Source: CAD feature listing. Evaluate the final solid. Frame: model axes, mm. Face numbers are marked on the shaded views. Coordinates: 2 decimals unless noted, no trailing zeros. Order: outer loops, then holes, each group sorted by start corner. A loop starts at its lowest first (then second) coordinate and runs counter-clockwise, first axis right, second up.
Autodesk Inventor part; units mm, degrees
ref_plane "YZ Plane" through (0, 0, 0) normal (1, 0, 0) x (0, 1, 0)
ref_plane "XZ Plane" through (0, 0, 0) normal (0, 1, 0) x (-1, 0, 0)
ref_plane "XY Plane" through (0, 0, 0) normal (0, 0, 1) x (1, 0, 0)
sketch "Sketch1" plane through (0, 0, 0) normal (0, 1, 0) x (-1, 0, 0)
  line L0 (-46.75, 58.25) -> (46.75, 58.25)
  line L1 (46.75, 58.25) -> (46.75, -58.25)
  line L2 (46.75, -58.25) -> (-46.75, -58.25)
  line L3 (-46.75, -58.25) -> (-46.75, 58.25)
  line L4 (-46.75, 58.25) -> (46.75, -58.25) construction
  line L5 (46.75, 58.25) -> (-46.75, -58.25) construction
  point P0 (0, 0)
  dimension "d0" = 116.5
  dimension "d1" = 93.5
extrude "Extrusion1" add sketch "Sketch1" along normal blind 8
sketch "Sketch2" plane through (0, 8, 0) normal (0, 1, 0) x (1, 0, 0)
  line L0 (43.75, -55.25) -> (-43.75, -55.25)
  line L1 (-43.75, -55.25) -> (-43.75, 55.25)
  line L2 (-43.75, 55.25) -> (43.75, 55.25)
  line L3 (43.75, 55.25) -> (43.75, -55.25)
  line L4 (43.75, -55.25) -> (-43.75, 55.25) construction
  line L5 (-43.75, -55.25) -> (43.75, 55.25) construction
  point P0 (0, 0)
  dimension "d4" = 110.5
  dimension "d5" = 87.5
extrude "Extrusion2" cut sketch "Sketch2" against normal blind 1.6
sketch "Sketch3" plane through (0, 6.4, 0) normal (0, 1, 0) x (1, 0, 0)
  line L0 (42.75, -54.25) -> (-42.75, -54.25)
  line L1 (-42.75, -54.25) -> (-42.75, 54.25)
  line L2 (-42.75, 54.25) -> (42.75, 54.25)
  line L3 (42.75, 54.25) -> (42.75, -54.25)
  line L4 (42.75, -54.25) -> (-42.75, 54.25) construction
  line L5 (-42.75, -54.25) -> (42.75, 54.25) construction
  point P0 (0, 0)
  dimension "d8" = 108.5
  dimension "d9" = 85.5
extrude "Extrusion3" cut sketch "Sketch3" against normal blind 4
sketch "Sketch4" plane through (0, 2.4, 0) normal (0, 1, 0) x (1, 0, 0)
  circle A0 centre (-39.5, -51) radius 4.75
  circle A1 centre (-39.5, 51) radius 4.75
  line L0 (42.75, -54.25) -> (-42.75, -54.25)
  circle A2 centre (39.5, -51) radius 4.75
  line L1 (42.75, 54.25) -> (42.75, -54.25)
  circle A3 centre (39.5, 51) radius 4.75
  line L2 (-42.75, -54.25) -> (-42.75, 54.25)
  line L3 (-43.75, -55.25) -> (-43.75, 55.25)
  line L4 (-43.75, 55.25) -> (43.75, 55.25)
  line L5 (43.75, -55.25) -> (-43.75, -55.25)
  point P0 (0, 0)
  point P1 (-42.75, 54.25)
  point P2 (-42.75, -47.5359)
  point P3 (-36.0359, -54.25)
  point P4 (42.75, -47.5359)
  point P5 (36.0359, -54.25)
  point P6 (41, 55.25)
  point P7 (41, -55.25)
  point P8 (-41, -55.25)
  point P9 (-41, 55.25)
  dimension "d12" = 9.5
  dimension "d13" = 9.5
  dimension "d14" = 102
  dimension "d17" = 9.5
  dimension "d20" = 79
  dimension "d21" = 9.5
  dimension "d22" = 102
  dimension "d23" = 79
  dimension "d42" = 4.25
  dimension "d43" = 4.25
  dimension "d44" = 4.25
  dimension "d45" = 4.25
extrude "Extrusion4" add sketch "Sketch4" along normal blind 4 contours A0 L0 L2 | L2 L0 A0 L5 L3 | L3 A0 | A1 L3 L4 | A0 L5 | A2 L1 L0 | L0 L1 A2 L5 | A1 L3 | L5 A2 | L4 A1 | A3 L4 | A3 L4 picked at (-38.9284, 52.0845)
sketch "Sketch5" plane through (0, 6.4, 0) normal (0, 1, 0) x (1, 0, 0)
  arc A0 (-36.0359, -54.25) -> (-42.75, -47.5359) centre (-39.5, -51) ccw
  circle A1 centre (-39.5, -51) radius 1.5
  arc A2 (-42.75, 47.5359) -> (-36.0359, 54.25) centre (-39.5, 51) ccw
  circle A3 centre (-39.5, 51) radius 1.5
  arc A4 (36.0359, 54.25) -> (42.75, 47.5359) centre (39.5, 51) ccw
  circle A5 centre (39.5, 51) radius 1.5
  arc A6 (42.75, -47.5359) -> (36.0359, -54.25) centre (39.5, -51) ccw
  circle A7 centre (39.5, -51) radius 1.5
  point P0 (0, 0)
  point P1 (-41.8318, -54.25)
  dimension "d27" = 3
  dimension "d28" = 3
  dimension "d29" = 3
  dimension "d30" = 3
extrude "Extrusion5" cut sketch "Sketch5" against normal blind 4
fillet "Fillet1" radius 1.5 4 edges at (-43.75, 7.2, 55.25) (-43.75, 7.2, -55.25) (43.75, 7.2, 55.25) (43.75, 7.2, -55.25)
sketch "Sketch6" plane through (0, 8, 0) normal (0, 1, 0) x (1, 0, 0)
  line L0 (45.25, -56.75) -> (-45.25, -56.75)
  line L1 (-45.25, -56.75) -> (-45.25, 56.75)
  line L2 (-45.25, 56.75) -> (45.25, 56.75)
  line L3 (45.25, 56.75) -> (45.25, -56.75)
  line L4 (45.25, -56.75) -> (-45.25, 56.75) construction
  line L5 (-45.25, -56.75) -> (45.25, 56.75) construction
  line L6 (50, -69.25) -> (-50, -69.25)
  line L7 (-50, -69.25) -> (-50, 69.25)
  line L8 (-50, 69.25) -> (50, 69.25)
  line L9 (50, 69.25) -> (50, -69.25)
  line L10 (50, -69.25) -> (-50, 69.25) construction
  line L11 (-50, -69.25) -> (50, 69.25) construction
  point P0 (0, 0)
  dimension "d35" = 113.5
  dimension "d36" = 90.5
  dimension "d37" = 138.5
  dimension "d38" = 100
extrude "Extrusion6" cut sketch "Sketch6" against normal blind 6
fillet "Fillet3" radius 1.5 8 edges at (45.25, 5, 56.75) (46.75, 1, 58.25) (45.25, 5, -56.75) (46.75, 1, -58.25) (-45.25, 5, -56.75) (-46.75, 1, -58.25) (-45.25, 5, 56.75) (-46.75, 1, 58.25)
properties part number "BoardMount"
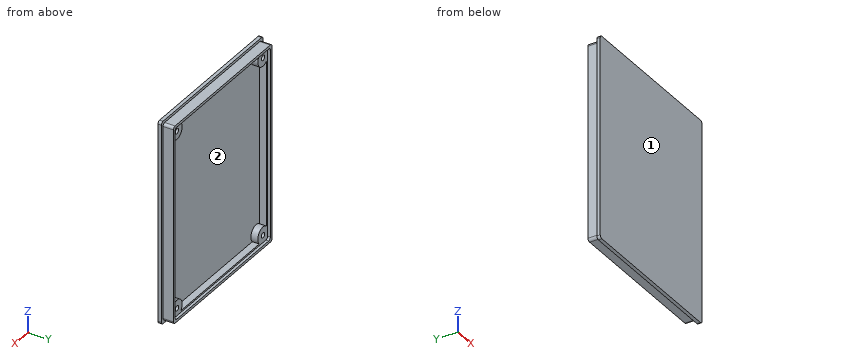
1. Contact query for flat-ended pins moving along their axis: P1, Ø3, axis at y = 6.5, z = 23, coming from the +X side; P2, Ø1.8, axis at x = -39.5, z = 51, coming from the +Y side; P3, Ø1, axis at x = 32, y = 5.5, coming from the -Z side. Output: stop coordinate, or through.
2. Section query B-B, the plane x = -39.5. Output: boundary loops of the cut face in (y, z), plus the area to 3 significant figures.
3. Section query D-D, the plane x = -10. Output: boundary loops of the cut face in (y, z).
4. Material intervals for line 1 along X through (y, z) = (4.4, -51); line 2 along Z through (x, y) = (-39.5, 3.6); line 3 along Z through (x, y) = (-3.5, 4), sorted ascending.
5. Draft query along X for the marked faces 1 and 2. Return one class per face: +X half, -X half, draft (parallel to the pull), parting line (faces both ways), or undercut.
6. Section query A-A, the plane z = -12.5. Output: boundary loops of the cut face in (x, y).
7. Section query C-C, the plane z = -51. Output: boundary loops of the cut face in (x, y), plus the area to 3 significant figures.
Answer key:
1. P1: stops at x = 45.25
1. P2: stops at y = 2.4
1. P3: stops at z = -56.75
2. outline: (0, -58.25) - (2, -58.25) - (2, -56.75) - (8, -56.75) - (8, -55.25) - (6.4, -55.25) - (6.4, -52.5) - (2.4, -52.5) - (2.4, -49.5) - (6.4, -49.5) - (6.4, -46.25) - (2.4, -46.25) - (2.4, 46.25) - (6.4, 46.25) - (6.4, 49.5) - (2.4, 49.5) - (2.4, 52.5) - (6.4, 52.5) - (6.4, 55.25) - (8, 55.25) - (8, 56.75) - (2, 56.75) - (2, 58.25) - (0, 58.25) - close
2. area: 343 mm2
3. outline: (0, -58.25) - (2, -58.25) - (2, -56.75) - (8, -56.75) - (8, -55.25) - (6.4, -55.25) - (6.4, -54.25) - (2.4, -54.25) - (2.4, 54.25) - (6.4, 54.25) - (6.4, 55.25) - (8, 55.25) - (8, 56.75) - (2, 56.75) - (2, 58.25) - (0, 58.25) - close
4. line 1: x = -45.25 to -41, -38 to -34.75, 34.75 to 38, 41 to 45.25
4. line 2: z = -56.75 to -52.5, -49.5 to -46.25, 46.25 to 49.5, 52.5 to 56.75
4. line 3: z = -56.75 to -54.25, 54.25 to 56.75
5. face 1: draft
5. face 2: undercut
6. outline: (-46.75, 0) - (46.75, 0) - (46.75, 2) - (45.25, 2) - (45.25, 8) - (43.75, 8) - (43.75, 6.4) - (42.75, 6.4) - (42.75, 2.4) - (-42.75, 2.4) - (-42.75, 6.4) - (-43.75, 6.4) - (-43.75, 8) - (-45.25, 8) - (-45.25, 2) - (-46.75, 2) - close
7. outline: (-46.75, 0) - (46.75, 0) - (46.75, 2) - (45.25, 2) - (45.25, 8) - (43.75, 8) - (43.75, 6.4) - (41, 6.4) - (41, 2.4) - (38, 2.4) - (38, 6.4) - (34.75, 6.4) - (34.75, 2.4) - (-34.75, 2.4) - (-34.75, 6.4) - (-38, 6.4) - (-38, 2.4) - (-41, 2.4) - (-41, 6.4) - (-43.75, 6.4) - (-43.75, 8) - (-45.25, 8) - (-45.25, 2) - (-46.75, 2) - close
7. area: 288 mm2
